Could you check a few things on this model? Use its own coordinates, in mm. Give positions to 0.01 mm unless a question says otherwise; leave off trailing zeros. Loops run counter-clockwise (first coordinate to the right, second up) from the corner with the lowest first, then second, coordinate; pieces in that order, holes last. Notation, with made-up numbers: M -1.5,80 L 37.5,80 A25 cw 37.5,101 Z; hole C 10.5,40.25 d7. An arc over 180 degrees is marked long. Write each question's results on one line, items separated by ' | '. Start each with the question number.
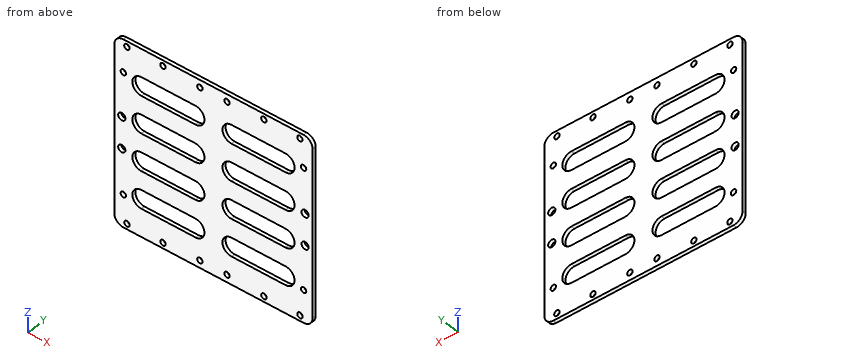
from build123d import *

# Parameters (mm, degrees)
SKETCH_1_W             = 110
SKETCH_1_H             = 100
SKETCH_1_R             = 1.5
SKETCH_1_R_2           = 2
EXTRUDE_1_DEPTH        = 2
FILLET_1_R             = 5
CUT_EXTRUDE_1903_DEPTH = 10
SKETCH_3_R             = 1.5
CUT_EXTRUDE_2113_DEPTH = 10
SKETCH_4_R             = 1.5
CUT_EXTRUDE_2323_DEPTH = 10


with BuildPart() as part:
    # 草图1 → 凸台-拉伸1 (new body)
    with BuildSketch(Plane(origin=(0, 0, 0), x_dir=(1, 0, 0), z_dir=(0, 1, 0))):
        Rectangle(SKETCH_1_W, SKETCH_1_H)
        with Locations(Location((-48, -47, 0), (0, 0, 270))):
            Circle(SKETCH_1_R, mode=Mode.SUBTRACT)
        with Locations(Location((-28, -47, 0), (0, 0, 270))):
            Circle(SKETCH_1_R, mode=Mode.SUBTRACT)
        with Locations(Location((-50.854561817, 8.5, 0), (0, 0, 270))):
            Circle(SKETCH_1_R_2, mode=Mode.SUBTRACT)
        with Locations(Location((-50.854561817, -8.5, 0), (0, 0, 270))):
            Circle(SKETCH_1_R_2, mode=Mode.SUBTRACT)
        with Locations(Location((-28, 47, 0), (0, 0, 270))):
            Circle(SKETCH_1_R, mode=Mode.SUBTRACT)
        with Locations(Location((-48, 47, 0), (0, 0, 270))):
            Circle(SKETCH_1_R, mode=Mode.SUBTRACT)
        with Locations(Location((28, -47, 0), (0, 0, 270))):
            Circle(SKETCH_1_R, mode=Mode.SUBTRACT)
        with Locations(Location((48, -47, 0), (0, 0, 270))):
            Circle(SKETCH_1_R, mode=Mode.SUBTRACT)
        with Locations(Location((48, 47, 0), (0, 0, 270))):
            Circle(SKETCH_1_R, mode=Mode.SUBTRACT)
        with Locations(Location((28, 47, 0), (0, 0, 270))):
            Circle(SKETCH_1_R, mode=Mode.SUBTRACT)
        with Locations(Location((50.854561817, -8.5, 0), (0, 0, 270))):
            Circle(SKETCH_1_R_2, mode=Mode.SUBTRACT)
        with Locations(Location((50.854561817, 8.5, 0), (0, 0, 270))):
            Circle(SKETCH_1_R_2, mode=Mode.SUBTRACT)
    extrude(amount=EXTRUDE_1_DEPTH)

    # 圆角1
    fillet_1_edges = [part.edges().sort_by_distance(p)[0] for p in [
        (55, 1, -50),
        (55, 1, 50),
        (-55, 1, 50),
        (-55, 1, -50),
    ]]
    fillet(fillet_1_edges, radius=FILLET_1_R)

    # 草图2 → Cut-Extrude 1903 (cut)
    with BuildSketch(Plane(origin=(0, 2, 0), x_dir=(1, 0, 0), z_dir=(0, 1, 0))):
        with BuildLine():
            Line((-40, 35), (-10, 35))
            ThreePointArc((-10, 35), (-5, 30), (-10, 25))
            Line((-10, 25), (-40, 25))
            ThreePointArc((-40, 25), (-45, 30), (-40, 35))
        make_face()
        with BuildLine():
            Line((-40, 15), (-10, 15))
            ThreePointArc((-10, 15), (-5, 10), (-10, 5))
            Line((-10, 5), (-40, 5))
            ThreePointArc((-40, 5), (-45, 10), (-40, 15))
        make_face()
        with BuildLine():
            Line((-40, -5), (-10, -5))
            ThreePointArc((-10, -5), (-5, -10), (-10, -15))
            Line((-10, -15), (-40, -15))
            ThreePointArc((-40, -15), (-45, -10), (-40, -5))
        make_face()
        with BuildLine():
            Line((-40, -25), (-10, -25))
            ThreePointArc((-10, -25), (-5, -30), (-10, -35))
            Line((-10, -35), (-40, -35))
            ThreePointArc((-40, -35), (-45, -30), (-40, -25))
        make_face()
        with BuildLine():
            Line((40, 35), (10, 35))
            ThreePointArc((10, 35), (5, 30), (10, 25))
            Line((10, 25), (40, 25))
            ThreePointArc((40, 25), (45, 30), (40, 35))
        make_face()
        with BuildLine():
            Line((40, 15), (10, 15))
            ThreePointArc((10, 15), (5, 10), (10, 5))
            Line((10, 5), (40, 5))
            ThreePointArc((40, 5), (45, 10), (40, 15))
        make_face()
        with BuildLine():
            Line((40, -5), (10, -5))
            ThreePointArc((10, -5), (5, -10), (10, -15))
            Line((10, -15), (40, -15))
            ThreePointArc((40, -15), (45, -10), (40, -5))
        make_face()
        with BuildLine():
            Line((40, -25), (10, -25))
            ThreePointArc((10, -25), (5, -30), (10, -35))
            Line((10, -35), (40, -35))
            ThreePointArc((40, -35), (45, -30), (40, -25))
        make_face()
    extrude(amount=-CUT_EXTRUDE_1903_DEPTH, mode=Mode.SUBTRACT)

    # 草图3 → Cut-Extrude 2113 (cut)
    with BuildSketch(Plane(origin=(0, 2, 0), x_dir=(1, 0, 0), z_dir=(0, 1, 0))):
        with Locations(Location((-7.5, 46, 0), (0, 0, 270))):
            Circle(SKETCH_3_R)
        with Locations(Location((7.5, 46, 0), (0, 0, 270))):
            Circle(SKETCH_3_R)
        with Locations(Location((-7.5, -46, 0), (0, 0, 270))):
            Circle(SKETCH_3_R)
        with Locations(Location((7.5, -46, 0), (0, 0, 270))):
            Circle(SKETCH_3_R)
    extrude(amount=-CUT_EXTRUDE_2113_DEPTH, mode=Mode.SUBTRACT)

    # 草图4 → Cut-Extrude 2323 (cut)
    with BuildSketch(Plane(origin=(0, 2, 0), x_dir=(1, 0, 0), z_dir=(0, 1, 0))):
        with Locations(Location((-50, -32.5, 0), (0, 0, 270))):
            Circle(SKETCH_4_R)
        with Locations(Location((50, -32.5, 0), (0, 0, 270))):
            Circle(SKETCH_4_R)
        with Locations(Location((50, 32.5, 0), (0, 0, 270))):
            Circle(SKETCH_4_R)
        with Locations(Location((-50, 32.5, 0), (0, 0, 270))):
            Circle(SKETCH_4_R)
    extrude(amount=-CUT_EXTRUDE_2323_DEPTH, mode=Mode.SUBTRACT)


solid = part.part
1) If we section it at B-B on z = -32.5: Write out the boundary of the cut face in (x, y), plus the area to 3 significant figures.
2) If we section it at A-A on x = -14: Write out the boundary of the cut face in (y, z).
3) If we section it at D-D on y = 1.65: State how many separate pieces and enclosed holes the cut face has, plus the area to 3 significant figures.
4) If we section it at C-C on x = 7.5: Write out the boundary of the cut face in (y, z).
5) Please list where these lines run through material, in increasing order: line 1 (Z direction, x = -18, y = 0.55); line 2 (X direction, y = 0.2, z = -10); line 3 (X direction, y = 0.95, z = -32.5). Write a range as from..to.
Calculated:
1) outline: M -55,0 L -51.5,0 L -51.5,2 L -55,2 Z; M -48.5,0 L -44.33,0 L -44.33,2 L -48.5,2 Z; M -5.67,0 L 5.67,0 L 5.67,2 L -5.67,2 Z; M 44.33,0 L 48.5,0 L 48.5,2 L 44.33,2 Z; M 51.5,0 L 55,0 L 55,2 L 51.5,2 Z | area: 53.4 mm2
2) outline: M 0,-50 L 2,-50 L 2,-35 L 0,-35 Z; M 0,-25 L 2,-25 L 2,-15 L 0,-15 Z; M 0,-5 L 2,-5 L 2,5 L 0,5 Z; M 0,15 L 2,15 L 2,25 L 0,25 Z; M 0,35 L 2,35 L 2,50 L 0,50 Z
3) separate pieces: 1 | enclosed holes: 28 | area: 7,790 mm2
4) outline: M 0,-50 L 2,-50 L 2,-47.5 L 0,-47.5 Z; M 0,-44.5 L 2,-44.5 L 2,-34.33 L 0,-34.33 Z; M 0,-25.67 L 2,-25.67 L 2,-14.33 L 0,-14.33 Z; M 0,-5.67 L 2,-5.67 L 2,5.67 L 0,5.67 Z; M 0,14.33 L 2,14.33 L 2,25.67 L 0,25.67 Z; M 0,34.33 L 2,34.33 L 2,44.5 L 0,44.5 Z; M 0,47.5 L 2,47.5 L 2,50 L 0,50 Z
5) line 1: z = -50..-35, -25..-15, -5..5, 15..25, 35..50 | line 2: x = -55..-52.18, -49.53..-45, -5..5, 45..49.53, 52.18..55 | line 3: x = -55..-51.5, -48.5..-44.33, -5.67..5.67, 44.33..48.5, 51.5..55
